```python
from build123d import *

# Parameters (mm, degrees)
F0_W     = 152.4
F0_H     = 203.2
F1_DEPTH = 3.175
F3_DEPTH = 25.4
F4_W     = 50.8
F4_H     = 50.8
F5_DEPTH = 679.45
F6_R     = 2.54
F8_DEPTH = 12.7
F9_SIZE2 = 6.35
F9_SIZE  = 6.35
F10_SIZE = 6.35


with BuildPart() as f1:
    # F0 (on Top) → F1 (new body)
    with BuildSketch(Plane.XY):
        Rectangle(F0_W, F0_H)
    extrude(amount=F1_DEPTH)

    # F2 (on face) → F3 (cut)
    with BuildSketch(Plane.XY.offset(3.175)):
        with BuildLine():
            Line((-2.523452, 48.276548), (0, 50.8))
            Line((0, 50.8), (2.523452, 48.276548))
            ThreePointArc((2.523452, 48.276548), (3.297049, 49.434318), (3.5687, 50.8))
            ThreePointArc((3.5687, 50.8), (-1.365682, 54.097049), (-2.523452, 48.276548))
        make_face()
        with BuildLine():
            Line((2.523452, 48.276548), (0, 50.8))
            Line((0, 50.8), (-2.523452, 48.276548))
            ThreePointArc((-2.523452, 48.276548), (0, 47.2313), (2.523452, 48.276548))
        make_face()
        with BuildLine():
            Line((-50.8, 0), (-48.276548, 2.523452))
            ThreePointArc((-48.276548, 2.523452), (-54.3687, 0), (-48.276548, -2.523452))
            Line((-48.276548, -2.523452), (-50.8, 0))
        make_face()
        with BuildLine():
            ThreePointArc((-47.2313, 0), (-47.502951, 1.365682), (-48.276548, 2.523452))
            Line((-48.276548, 2.523452), (-50.8, 0))
            Line((-50.8, 0), (-48.276548, -2.523452))
            ThreePointArc((-48.276548, -2.523452), (-47.502951, -1.365682), (-47.2313, 0))
        make_face()
        with BuildLine():
            Line((50.8, 0), (48.276548, 2.523452))
            ThreePointArc((48.276548, 2.523452), (47.2313, 0), (48.276548, -2.523452))
            Line((48.276548, -2.523452), (50.8, 0))
        make_face()
        with BuildLine():
            ThreePointArc((54.3687, 0), (52.165682, 3.297049), (48.276548, 2.523452))
            Line((48.276548, 2.523452), (50.8, 0))
            Line((50.8, 0), (48.276548, -2.523452))
            ThreePointArc((48.276548, -2.523452), (52.165682, -3.297049), (54.3687, 0))
        make_face()
        with BuildLine():
            Line((0, -50.8), (2.523452, -48.276548))
            ThreePointArc((2.523452, -48.276548), (0, -47.2313), (-2.523452, -48.276548))
            Line((-2.523452, -48.276548), (0, -50.8))
        make_face()
        with BuildLine():
            ThreePointArc((3.5687, -50.8), (3.297049, -49.434318), (2.523452, -48.276548))
            Line((2.523452, -48.276548), (0, -50.8))
            Line((0, -50.8), (-2.523452, -48.276548))
            ThreePointArc((-2.523452, -48.276548), (-1.365682, -54.097049), (3.5687, -50.8))
        make_face()
        with BuildLine():
            ThreePointArc((-59.9313, -88.9), (-60.976548, -86.376548), (-63.5, -85.3313))
            Line((-63.5, -85.3313), (-63.5, -88.9))
            Line((-63.5, -88.9), (-59.9313, -88.9))
        make_face()
        with BuildLine():
            Line((-63.5, -88.9), (-63.5, -85.3313))
            ThreePointArc((-63.5, -85.3313), (-66.023452, -91.423452), (-59.9313, -88.9))
            Line((-59.9313, -88.9), (-63.5, -88.9))
        make_face()
        with BuildLine():
            Line((63.5, -88.9), (63.5, -85.3313))
            ThreePointArc((63.5, -85.3313), (60.976548, -86.376548), (59.9313, -88.9))
            Line((59.9313, -88.9), (63.5, -88.9))
        make_face()
        with BuildLine():
            ThreePointArc((67.0687, -88.9), (66.023452, -86.376548), (63.5, -85.3313))
            Line((63.5, -85.3313), (63.5, -88.9))
            Line((63.5, -88.9), (59.9313, -88.9))
            ThreePointArc((59.9313, -88.9), (63.5, -92.4687), (67.0687, -88.9))
        make_face()
        with BuildLine():
            ThreePointArc((67.0687, 88.9), (63.5, 92.4687), (59.9313, 88.9))
            Line((59.9313, 88.9), (63.5, 88.9))
            Line((63.5, 88.9), (63.5, 85.3313))
            ThreePointArc((63.5, 85.3313), (66.023452, 86.376548), (67.0687, 88.9))
        make_face()
        with BuildLine():
            Line((63.5, 88.9), (59.9313, 88.9))
            ThreePointArc((59.9313, 88.9), (60.976548, 86.376548), (63.5, 85.3313))
            Line((63.5, 85.3313), (63.5, 88.9))
        make_face()
        with BuildLine():
            Line((-63.5, 88.9), (-59.9313, 88.9))
            ThreePointArc((-59.9313, 88.9), (-66.023452, 91.423452), (-63.5, 85.3313))
            Line((-63.5, 85.3313), (-63.5, 88.9))
        make_face()
        with BuildLine():
            ThreePointArc((-63.5, 85.3313), (-60.976548, 86.376548), (-59.9313, 88.9))
            Line((-59.9313, 88.9), (-63.5, 88.9))
            Line((-63.5, 88.9), (-63.5, 85.3313))
        make_face()
    extrude(amount=-F3_DEPTH, mode=Mode.SUBTRACT)

    # F4 (on face) → F5 (join)
    with BuildSketch(Plane(origin=(0, 0, 0), x_dir=(1, 0, 0), z_dir=(0, 0, -1))):
        Rectangle(F4_W, F4_H)
    extrude(amount=F5_DEPTH)

    # F6
    f6_edges = [f1.edges().sort_by_distance(p)[0] for p in [
        (-25.4, -25.4, -339.725),
        (25.4, -25.4, -339.725),
        (25.4, 25.4, -339.725),
        (-25.4, 25.4, -339.725),
    ]]
    fillet(f6_edges, radius=F6_R)

    # F7 (on face) → F8 (join)
    with BuildSketch(Plane(origin=(0, 0, -679.45), x_dir=(1, 0, 0), z_dir=(0, 0, -1))):
        with BuildLine():
            Line((25.4, 22.86), (25.4, 228.6))
            Line((25.4, 228.6), (-25.4, 228.6))
            Line((-25.4, 228.6), (-25.4, 22.86))
            ThreePointArc((-25.4, 22.86), (-24.656051, 24.656051), (-22.86, 25.4))
            Line((-22.86, 25.4), (22.86, 25.4))
            ThreePointArc((22.86, 25.4), (24.656051, 24.656051), (25.4, 22.86))
        make_face()
        with BuildLine():
            Line((25.4, -228.6), (25.4, -22.86))
            ThreePointArc((25.4, -22.86), (24.656051, -24.656051), (22.86, -25.4))
            Line((22.86, -25.4), (-22.86, -25.4))
            ThreePointArc((-22.86, -25.4), (-24.656051, -24.656051), (-25.4, -22.86))
            Line((-25.4, -22.86), (-25.4, -228.6))
            Line((-25.4, -228.6), (25.4, -228.6))
        make_face()
        with BuildLine():
            Line((25.4, -22.86), (25.4, 22.86))
            ThreePointArc((25.4, 22.86), (24.656051, 24.656051), (22.86, 25.4))
            Line((22.86, 25.4), (-22.86, 25.4))
            ThreePointArc((-22.86, 25.4), (-24.656051, 24.656051), (-25.4, 22.86))
            Line((-25.4, 22.86), (-25.4, -22.86))
            ThreePointArc((-25.4, -22.86), (-24.656051, -24.656051), (-22.86, -25.4))
            Line((-22.86, -25.4), (22.86, -25.4))
            ThreePointArc((22.86, -25.4), (24.656051, -24.656051), (25.4, -22.86))
        make_face()
    extrude(amount=F8_DEPTH)

    # F9
    f9_edges = [f1.edges().sort_by_distance(p)[0] for p in [
        (0, -228.6, -679.45),
        (0, 228.6, -679.45),
    ]]
    chamfer(f9_edges, length=F9_SIZE, length2=F9_SIZE2)

    # F10
    f10_edges = [f1.edges().sort_by_distance(p)[0] for p in [
        (25.4, -122.555, -679.45),
        (25.4, 122.555, -679.45),
        (-25.4, -122.555, -679.45),
        (-25.4, 122.555, -679.45),
    ]]
    chamfer(f10_edges, length=F10_SIZE)


solid = f1.part
```
The model under review builds one solid part; all positions refer to its coordinate system, in mm. A direction names the side the tool comes from. Round coordinates to 2 decimals unless told otherwise and drop trailing zeros. Loops run counter-clockwise (first coordinate to the right, second up) from the corner with the lowest first, then second, coordinate; pieces in that order, holes last. Notation, with made-up numbers: (-26.75, 79.5) -> (1.25, 79.5) arc R21 ccw to (1.25, 117.5) -> close; hole circle Ø2 at (28, -28). An arc over 180 degrees is marked (long way). Answer in a Markdown table with one row per item.
1) For pin 1 Ø2.5 at (x, z) = (11.5, 1) entering from -Y; pin 2 Ø2 at (x, z) = (24, -321) entering from -Y; pin 3 Ø10 at (y, z) = (13.5, -476.5) entering from +X; pin 4 Ø5.5 at (x, y) = (-63.5, 88.9) entering from +Z, all flat-tipped, find the tip position at first contact; note any pin that passes through.
Taken from the geometry:
| item | result |
|---|---|
| pin 1 | stops at y = -101.6 |
| pin 2 | stops at y = -25.4 |
| pin 3 | stops at x = 25.4 |
| pin 4 | passes through |
2) Consider section B-B, the plane z = -508.5. Write out the cut boundary in (x, y).
Taken from the geometry:
| item | result |
|---|---|
| outline | (-25.4, -22.86) arc R2.54 ccw to (-22.86, -25.4) -> (22.86, -25.4) arc R2.54 ccw to (25.4, -22.86) -> (25.4, 22.86) arc R2.54 ccw to (22.86, 25.4) -> (-22.86, 25.4) arc R2.54 ccw to (-25.4, 22.86) -> close |
3) Draft analysis for pull direction Z (two halves, no side actions). For faces 1 (the flat face through (0, -3, -692.15)), 2 (the flat face through (-1, 1, 3.175)), 3 (the flat face through (0, 25.4, -337)), 4 (the flat face through (0, -25.4, -337)), state which applies: pulls with the +Z half, pulls with the -Z half, needs draft (parallel to the pull), parting line crosses it, or undercut.
Taken from the geometry:
| item | result |
|---|---|
| face 1 | pulls with the -Z half |
| face 2 | pulls with the +Z half |
| face 3 | undercut |
| face 4 | undercut |
4) Wall thickness on line 1 along Y through (x, z) = (0, 2.25); line 2 along X through (y, z) = (-88.9, 1.05); line 3 along Y through (x, z) = (-50, 1): over which ranges is each line inside the solid? List them lowest first.
Taken from the geometry:
| item | result |
|---|---|
| line 1 | y = -101.6 to -54.37, -47.23 to 47.23, 54.37 to 101.6 |
| line 2 | x = -76.2 to -67.07, -59.93 to 59.93, 67.07 to 76.2 |
| line 3 | y = -101.6 to -3.48, 3.48 to 101.6 |
5) Consider section C-C, the plane x = -32.5. Write out the cut boundary in (y, z) (3 decimals), plus the area to 3 significant figures.
Taken from the geometry:
| item | result |
|---|---|
| outline | (-101.6, 0) -> (101.6, 0) -> (101.6, 3.175) -> (-101.6, 3.175) -> close |
| area | 645 mm² |
6) Tool access review of faces 5 (the flat face through (-25.4, -1, -344)), 6 (the flat face through (0, 122, -679.45)), 7 (the flat face through (25.4, 1, -344)): name each direction out of +Z, -Z, +X, -X, +Y, -Y from which nothing blocks a thin tool from reaching the whole face with its end or side.
Taken from the geometry:
| item | result |
|---|---|
| face 5 | -Z, -X, +Y, -Y |
| face 6 | +X, -X, +Y |
| face 7 | -Z, +X, +Y, -Y |
7) Consider section A-A, the plane y = -75. Write out the cut boundary in (x, z) (3 decimals), plus the area to 3 significant figures.
Taken from the geometry:
| item | result |
|---|---|
| outline | (-76.2, 0) -> (76.2, 0) -> (76.2, 3.175) -> (-76.2, 3.175) -> close; (-25.4, -692.15) -> (25.4, -692.15) -> (25.4, -685.8) -> (19.05, -679.45) -> (-19.05, -679.45) -> (-25.4, -685.8) -> close |
| area | 1,090 mm² |
